Verification items for this drawing (mm, ordinates from the low corner). A direction names the side the tool comes from. Give positions to 0.01 mm unless a question says otherwise; leave off trailing zeros. Write each loop counter-clockwise with the first axis right and the second up, starting at its lowest first coordinate (ties: lowest second). Pieces come first, ordered by that corner, then holes. Notation, with made-up numbers: (14.5, 18.25) -> (48.5, 18.25) arc R8 ccw to (48.5, 27.25) -> close; hole circle Ø8 at (83.5, 46). An arc over 180 degrees is marked (long way). Write item = value, one per line.
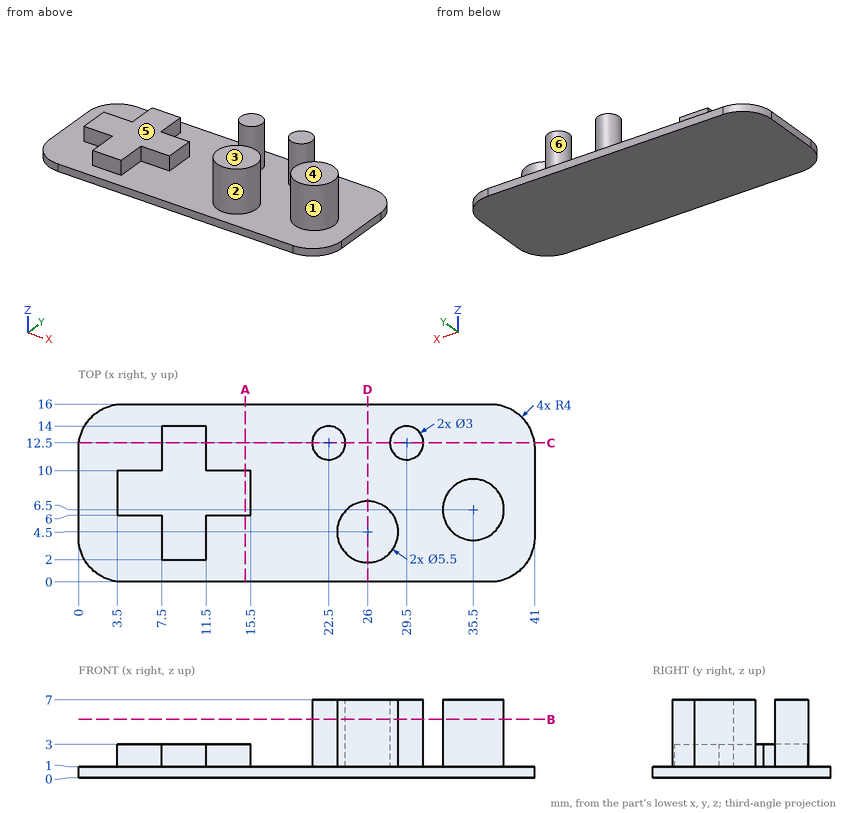
Item 1: Sectioned sample at A-A on x = 15. Record the cut outline in (y, z).
Response values:
outline = (0, 0) -> (16, 0) -> (16, 1) -> (10, 1) -> (10, 3) -> (6, 3) -> (6, 1) -> (0, 1) -> close
Item 2: Set-up check for the marked faces 4, 5 and 6: record each of +Z, -Z, +X, -X, +Y, -Y from which the full face is reachable in a straight line by a thin tool's end or side.
Response values:
face_4 = +Z, +X, -X, +Y, -Y
face_5 = +Z, -X, +Y, -Y
face_6 = +Z
Item 3: Mould release check, pull along Y, two halves, no side actions. Record for the marked faces 1, 2 and 3: +Y half, -Y half, draft (parallel to the pull), parting line (faces both ways), or undercut.
Response values:
face_1 = parting line
face_2 = undercut
face_3 = draft
Item 4: Sectioned sample at C-C on y = 12.5. Record the cut outline in (x, z), then the cut area to 3 significant figures.
Response values:
outline = (0.03, 0) -> (40.97, 0) -> (40.97, 1) -> (31, 1) -> (31, 7) -> (28, 7) -> (28, 1) -> (24, 1) -> (24, 7) -> (21, 7) -> (21, 1) -> (11.5, 1) -> (11.5, 3) -> (7.5, 3) -> (7.5, 1) -> (0.03, 1) -> close
area = 84.9 mm^2
Item 5: Sectioned sample at D-D on x = 26. Record the cut outline in (y, z), then the cut area to 3 significant figures.
Response values:
outline = (0, 0) -> (16, 0) -> (16, 1) -> (7.25, 1) -> (7.25, 7) -> (1.75, 7) -> (1.75, 1) -> (0, 1) -> close
area = 49.0 mm^2
Item 6: Material ranges on line 1 (Z direction, x = 7, y = 6.5); line 2 (Z direction, x = 35, y = 11); line 3 (X direction, y = 5.25, z = 1.5), recorded low to high.
Response values:
line_1 = 0 to 3
line_2 = 0 to 1
line_3 = 7.5 to 11.5, 23.35 to 28.65, 33.05 to 37.95
Item 7: Sectioned sample at B-B on z = 5.25. Record the cut outline in (x, y).
Response values:
outline = circle Ø3 at (22.5, 12.5); circle Ø5.5 at (26, 4.5); circle Ø3 at (29.5, 12.5); circle Ø5.5 at (35.5, 6.5)
Item 8: Go/stop test with flat-tipped pins: P1, Ø4, axis at x = 35.5, z = 6, coming from the -Y side; P2, Ø1, axis at y = 5, z = 2, coming from the -X side; P3, Ø1.6, axis at x = 6, z = 2, coming from the -Y side. Record where each tip stops, or that it passes through.
Response values:
P1 = 3.75
P2 = 7.5
P3 = 6
